For this review, use the dimensioned drawing (mm, ordinates from the lowest corner) and the shaded views. A direction names the side the tool comes from. Give positions to 0.01 mm unless a question says otherwise; leave off trailing zeros. Order: outer loops, then holes, each group sorted by start corner. A loop starts at its lowest first (then second) coordinate and runs counter-clockwise, first axis right, second up. Notation, with made-up numbers: M -16,88 L -9,88 A18 ccw -9,116 Z; hole C 83.25,54 d2. An arc over 180 degrees is marked long. One line per question, with ' | ' between items. Start each with the question number.
1. We need section C-C on y = 18. Write out the cut boundary in (x, z).
2. We need section B-B on x = 77. Write out the cut boundary in (y, z), then the cut area to 3 significant figures.
3. Insertion check: P1, Ø8, axis at x = 51.5, y = 78.5, coming from the -Z side; P2, Ø1.3, axis at y = 8.5, z = 1, coming from the -X side; P3, Ø16.5, axis at y = 103, z = 32.5, coming from the -X side. Each pin has a flat end and moves straight along its axis. Give the tip position at first contact, or say it passes through.
4. For the marked faces 1 and 2, list the 3-axis set-ups (+Z, -Z, +X, -X, +Y, -Y) from which the entire face can be reached by the end or side of a thin tool; tool diameter is ignored.
5. We need section D-D on x = 53.5. Write out the cut boundary in (y, z), then the cut area to 3 significant figures.
6. We need section A-A on z = 32.5. Write out the cut boundary in (x, y).
7. Wall thickness on L1, parallel to X at y = 18, z = 36; L2, parallel to Y at x = 5, z = 1; L3, parallel to Y at x = 59, z = 20.5: over which ranges is each line inside the solid? List them lowest first.
8. The part is to be moulded in two halves that separate along Y. For the marked faces 3, 4, 5 and 6, say which applies: +Y half, -Y half, draft (parallel to the pull), parting line (faces both ways), or undercut.
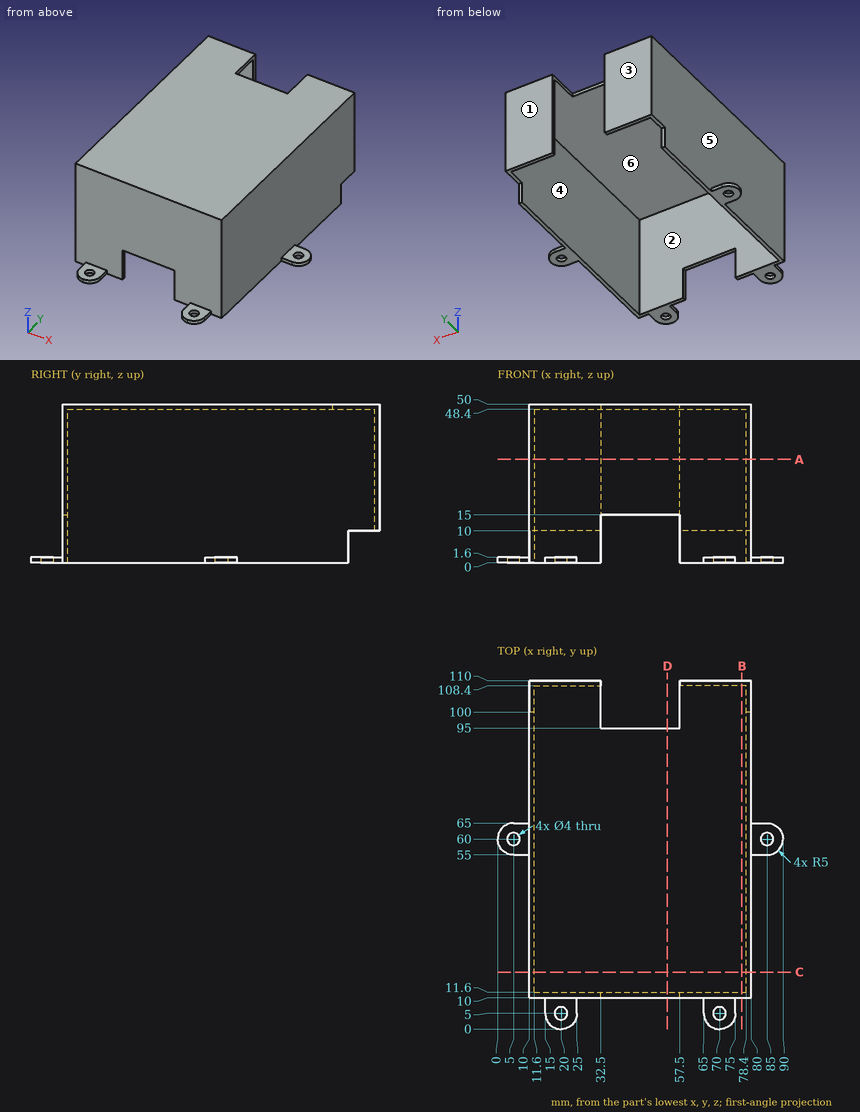
Entries:
1) outline: M 10,0 L 11.6,0 L 11.6,48.4 L 78.4,48.4 L 78.4,0 L 80,0 L 80,50 L 10,50 Z
2) outline: M 10,0 L 11.6,0 L 11.6,48.4 L 108.4,48.4 L 108.4,10 L 110,10 L 110,50 L 10,50 Z | area: 299 mm^2
3) P1: stops at z = 48.4 | P2: stops at x = 15 | P3: stops at x = 10
4) face 1: +Z, -Z, +X, -X, +Y | face 2: -Z
5) outline: M 10,15 L 11.6,15 L 11.6,48.4 L 95,48.4 L 95,50 L 10,50 Z | area: 189 mm^2
6) outline: M 10,10 L 80,10 L 80,110 L 57.5,110 L 57.5,108.4 L 78.4,108.4 L 78.4,11.6 L 11.6,11.6 L 11.6,108.4 L 32.5,108.4 L 32.5,110 L 10,110 Z
7) L1: x = 10 to 11.6, 78.4 to 80 | L2: y = 55 to 58, 62 to 65 | L3: y = 10 to 11.6, 108.4 to 110
8) face 3: +Y half | face 4: undercut | face 5: draft | face 6: undercut
